```python
from build123d import *

# Parameters (mm, degrees)
BOX_DEPTH                         = 9.25
BOX_DEPTH_BACK                    = 9.25
SKETCH1_W                         = 96
SKETCH1_H                         = 71
SKETCH2_W                         = 7.5
SKETCH2_H                         = 5
SWITCH_HOLE_DEPTH                 = 3
SKETCH4_W                         = 3
SKETCH4_H                         = 3
SWITCH_DEPTH                      = 5
SKETCH5_R                         = 2
WIRE_HOLE_DEPTH                   = 5
SKETCH7_W                         = 96
SKETCH7_H                         = 0.2
LID_INDICATOR_FRONT_DEPTH         = 1
SKETCH8_W                         = 70
SKETCH8_H                         = 0.2
LID_INDICATOR_LEFT_DEPTH          = 1
SKETCH9_W                         = 70
SKETCH9_H                         = 0.2
LID_INDICATOR_RIGHT_DEPTH         = 1
SKETCH10_W                        = 96
SKETCH10_H                        = 0.2
LID_INDICATOR_TOP_DEPTH           = 1
SKETCH11_W                        = 0.2
SKETCH11_H                        = 5.75
LID_INDICATOR_LEFT_SNIPPET_DEPTH  = 1
SKETCH12_W                        = 0.2
SKETCH12_H                        = 5.75
LID_INDICATOR_RIGHT_SNIPPET_DEPTH = 1
BOTTOM_ROUND_R                    = 3
TOP_ROUND_R                       = 3


with BuildPart() as part:
    # Sketch1 → Box (new, two sides: drawn at the far end of the back side and taken through both)
    with BuildSketch(Plane(origin=(0, 0, 0), x_dir=(1, 0, 0), z_dir=(0, 1, 0)).offset(-BOX_DEPTH_BACK)):
        Rectangle(SKETCH1_W, SKETCH1_H)
    extrude(amount=BOX_DEPTH + BOX_DEPTH_BACK)

    # Sketch2 → Switch Hole (cut)
    with BuildSketch(Plane.XY.offset(35.5)):
        with Locations((-35.25, 0)):
            Rectangle(SKETCH2_W, SKETCH2_H)
    extrude(amount=-SWITCH_HOLE_DEPTH, mode=Mode.SUBTRACT)

    # Sketch4 → Switch (add)
    with BuildSketch(Plane.XY.offset(32.5)):
        with Locations((-36.90464297, 0)):
            Rectangle(SKETCH4_W, SKETCH4_H)
    extrude(amount=SWITCH_DEPTH)

    # Sketch5 → Wire Hole (cut)
    with BuildSketch(Plane.XY.offset(35.5)):
        with Locations((-15.5, -6.25)):
            Circle(SKETCH5_R)
    extrude(amount=-WIRE_HOLE_DEPTH, mode=Mode.SUBTRACT)

    # Sketch7 → Lid Indicator Front (cut)
    with BuildSketch(Plane.XY.offset(35.5)):
        with Locations((0, 2.6)):
            Rectangle(SKETCH7_W, SKETCH7_H)
    extrude(amount=-LID_INDICATOR_FRONT_DEPTH, mode=Mode.SUBTRACT)

    # Sketch8 → Lid Indicator Left (cut)
    with BuildSketch(Plane.ZY.offset(48)):
        with Locations((0.5, 2.6)):
            Rectangle(SKETCH8_W, SKETCH8_H)
    extrude(amount=-LID_INDICATOR_LEFT_DEPTH, mode=Mode.SUBTRACT)

    # Sketch9 → Lid Indicator Right (cut)
    with BuildSketch(Plane(origin=(48, 0, 0), x_dir=(0, 0, -1), z_dir=(1, 0, 0))):
        with Locations((-0.5, 2.6)):
            Rectangle(SKETCH9_W, SKETCH9_H)
    extrude(amount=-LID_INDICATOR_RIGHT_DEPTH, mode=Mode.SUBTRACT)

    # Sketch10 → Lid Indicator Top (cut)
    with BuildSketch(Plane(origin=(0, 9.25, 0), x_dir=(1, 0, 0), z_dir=(0, 1, 0))):
        with Locations((0, 34.5)):
            Rectangle(SKETCH10_W, SKETCH10_H)
    extrude(amount=-LID_INDICATOR_TOP_DEPTH, mode=Mode.SUBTRACT)

    # Sketch11 → Lid Indicator Left Snippet (cut)
    with BuildSketch(Plane.ZY.offset(48)):
        with Locations((-34.5, 5.375)):
            Rectangle(SKETCH11_W, SKETCH11_H)
    extrude(amount=-LID_INDICATOR_LEFT_SNIPPET_DEPTH, mode=Mode.SUBTRACT)

    # Sketch12 → Lid Indicator Right Snippet (cut)
    with BuildSketch(Plane(origin=(48, 0, 0), x_dir=(0, 0, -1), z_dir=(1, 0, 0))):
        with Locations((34.5, 5.375)):
            Rectangle(SKETCH12_W, SKETCH12_H)
    extrude(amount=-LID_INDICATOR_RIGHT_SNIPPET_DEPTH, mode=Mode.SUBTRACT)

    # Bottom ROund
    bottom_round_edges = [part.edges().sort_by_distance(p)[0] for p in [
        (-48, -9.25, 0),
        (48, -9.25, 0),
    ]]
    fillet(bottom_round_edges, radius=BOTTOM_ROUND_R)

    # Top Round
    top_round_edges = [part.edges().sort_by_distance(p)[0] for p in [
        (48, 9.25, -35.05),
        (-48, 9.25, 0.55),
        (48, 9.25, 0.55),
        (-48, 9.25, -35.05),
    ]]
    fillet(top_round_edges, radius=TOP_ROUND_R)


solid = part.part
```
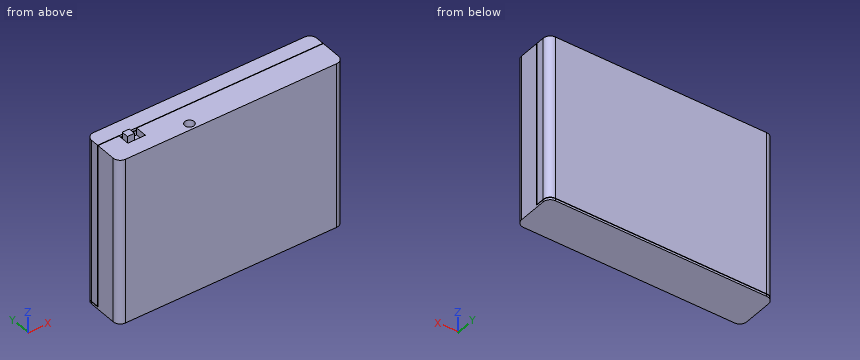
Could you check a few things on this model? Use its own coordinates, in mm. Round coordinates to 2 decimals unless told otherwise and drop trailing zeros. Write each loop counter-clockwise with the first axis right and the second up, starting at its lowest first coordinate (ties: lowest second). Pieces come first, ordered by that corner, then holes. Notation, with made-up numbers: M 87.5,82.25 L 141.5,82.25 A26 ccw 141.5,117.25 Z; hole C 40.25,-8 d11. An arc over 180 degrees is marked long. Answer in a Markdown table with one row per item. Add a question column.
Q1. Will these pins go through, and if not, where does the flat tip stop? pin 1 Ø4 at (x, y) = (12.5, -7.5) entering from +Z; pin 2 Ø1.2 at (x, y) = (-16.5, -5.5) entering from +Z.
Q2. Imagine slicing it at B-B (x = -15.5). Please give me the cut outline in (y, z).
Q3. If I drill on line 1 (Y direction, x = -15.5, z = 32.8); line 2 (Z direction, x = 16, y = -7.5); line 3 (X direction, y = -6.5, z = -3.5), over which ranges is the centre line in solid material (lowest first)? Write a range as from..to.
Q4. Imagine slicing it at A-A (x = -30). Please give me the cut outline in (y, z), then the cut area to 3 significant figures.
Values:
| question | item | result |
|---|---|---|
| 1 | pin 1 | z = 35.5 |
| 1 | pin 2 | z = 30.5 |
| 2 | outline | M -9.25,-35.5 L 9.25,-35.5 L 9.25,-34.6 L 8.25,-34.6 L 8.25,-34.4 L 9.25,-34.4 L 9.25,35.5 L 2.7,35.5 L 2.7,34.5 L 2.5,34.5 L 2.5,35.5 L -4.25,35.5 L -4.25,30.5 L -8.25,30.5 L -8.25,35.5 L -9.25,35.5 Z |
| 3 | line 1 | -9.25..-8.25, -4.25..9.25 |
| 3 | line 2 | -35.5..35.5 |
| 3 | line 3 | -47.99..47.99 |
| 4 | outline | M -9.25,-35.5 L 9.25,-35.5 L 9.25,-34.6 L 8.25,-34.6 L 8.25,-34.4 L 9.25,-34.4 L 9.25,35.5 L 2.7,35.5 L 2.7,34.5 L 2.5,34.5 L 2.5,35.5 L -9.25,35.5 Z |
| 4 | area | 1,310 mm^2 |
